Can you work these out from the model? Positions are in its coordinate system, mm. Coordinates: 2 decimals unless noted, no trailing zeros. Order: outer loops, then holes, each group sorted by start corner. A loop starts at its lowest first (then second) coordinate and runs counter-clockwise, first axis right, second up.
```python
from build123d import *

# Parameters (mm, degrees)
SKETCH1_R           = 31.525
BOSS_EXTRUDE1_DEPTH = 52.86
SKETCH2_R           = 5
BOSS_EXTRUDE2_DEPTH = 30.28
SKETCH3_R           = 2
CUT_EXTRUDE1_DEPTH  = 3
CIRPATTERN11_COUNT  = 4


with BuildPart() as part:
    # Sketch1 → Boss-Extrude1 (new body)
    with BuildSketch(Plane(origin=(0, 0, 0), x_dir=(1, 0, 0), z_dir=(0, 1, 0))):
        with Locations(Location((0, 0, 0), (0, 0, 270))):
            Circle(SKETCH1_R)
    extrude(amount=BOSS_EXTRUDE1_DEPTH)

    # Sketch2 → Boss-Extrude2 (add)
    with BuildSketch(Plane(origin=(0, 52.86, 0), x_dir=(1, 0, 0), z_dir=(0, 1, 0))):
        with Locations(Location((0, 0, 0), (0, 0, 270))):
            Circle(SKETCH2_R)
    extrude(amount=BOSS_EXTRUDE2_DEPTH)

    # Sketch3 → Cut-Extrude1 (cut)
    with BuildSketch(Plane(origin=(0, 52.86, 0), x_dir=(1, 0, 0), z_dir=(0, 1, 0))):
        with Locations(Location((0, 14.7, 0), (0, 0, 270))):
            Circle(SKETCH3_R)
        with Locations(Location((0, 21.94, 0), (0, 0, 270))):
            Circle(SKETCH3_R)
    cut_extrude1 = extrude(amount=-CUT_EXTRUDE1_DEPTH, mode=Mode.SUBTRACT)

    # CirPattern11: Cut-Extrude1 ×4 about axis
    cirpattern11_axis = Axis((0, 0, 0), (0, 1, 0))
    for i in range(1, CIRPATTERN11_COUNT):
        add(cut_extrude1.rotate(cirpattern11_axis, i * 360 / CIRPATTERN11_COUNT), mode=Mode.SUBTRACT)


solid = part.part
```
1. Imagine slicing it at B-B on z = -14.7. Please give me the cut outline in (x, y), then the cut area to 3 significant figures.
Completed:
outline: (-27.89, 0) - (27.89, 0) - (27.89, 52.86) - (2, 52.86) - (2, 49.86) - (-2, 49.86) - (-2, 52.86) - (-27.89, 52.86) - close
area: 2,940 mm2
2. Imagine slicing it at A-A on x = 0. Please give me the cut outline in (y, z) (3 decimals).
Completed:
outline: (0, -31.525) - (52.86, -31.525) - (52.86, -23.94) - (49.86, -23.94) - (49.86, -19.94) - (52.86, -19.94) - (52.86, -16.7) - (49.86, -16.7) - (49.86, -12.7) - (52.86, -12.7) - (52.86, -5) - (83.14, -5) - (83.14, 5) - (52.86, 5) - (52.86, 12.7) - (49.86, 12.7) - (49.86, 16.7) - (52.86, 16.7) - (52.86, 19.94) - (49.86, 19.94) - (49.86, 23.94) - (52.86, 23.94) - (52.86, 31.525) - (0, 31.525) - close
3. Imagine slicing it at C-C on y = 61.5. Please give me the cut outline in (x, z), then the cut area to 3 significant figures.
Completed:
outline: circle Ø10 at (0, 0)
area: 78.5 mm2
4. I'm going to push flat-ended pins straight in: pin 1 (5 mm diameter, centred on x = 0, z = -21.94, fed in from +Y); pin 2 (2 mm diameter, centred on x = 0.5, z = 21.5, fed in from +Y); pin 3 (10 mm diameter, centred on x = 13.5, y = 17.5, fed in from -Z). Where does each tip first touch, or does it pass through?
Completed:
pin 1: stops at y = 52.86
pin 2: stops at y = 49.86
pin 3: stops at z = -30.36
5. Please list where these lines run through material, in increasing order: probe 1 along Y at (x, z) = (-9, 10.5); probe 2 along X at (y, z) = (51.25, -21.94); probe 3 along X at (y, z) = (4.5, 20.5).
Completed:
probe 1: y = 0 to 52.86
probe 2: x = -22.64 to -2, 2 to 22.64
probe 3: x = -23.95 to 23.95
6. Imagine slicing it at D-D on x = -14.5. Please give me the cut outline in (y, z).
Completed:
outline: (0, -27.99) - (52.86, -27.99) - (52.86, -1.99) - (49.86, -1.99) - (49.86, 1.99) - (52.86, 1.99) - (52.86, 27.99) - (0, 27.99) - close
7. Thinking about a two-plate mould opening in Z: for faces 1 (the flat face through (0, 83.14, 0)), 2 (the cylindrical face through (-19.18, 26.06, -25.02)), 3 (the cylindrical face through (0.088, 51.381, -23.938)), which applies, pulls with the +Z half, pulls with the -Z half, needs draft (parallel to the pull), parting line crosses it, or undercut?
Completed:
face 1: needs draft
face 2: parting line crosses it
face 3: undercut
